For this review, take the finished solid that the model builds, in its own axes (mm). Face numbers are marked on the shaded views. A direction names the side the tool comes from. Give positions to 0.01 mm unless a question says otherwise; leave off trailing zeros. Order: outer loops, then holes, each group sorted by start corner. A loop starts at its lowest first (then second) coordinate and runs counter-clockwise, first axis right, second up.
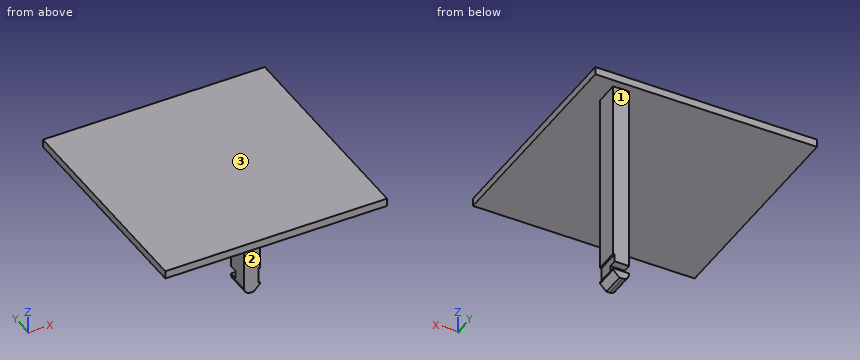
from build123d import *

# Parameters (mm, degrees)
F1_W      = 177.8
F1_H      = 177.8
F2_DEPTH  = 6.35
F3_W      = 12.7
F3_H      = 19.05
F4_DEPTH  = 165.1
F5_W      = 19.05
F5_H      = 12.7
F6_DEPTH  = 1.27
F7_SIZE   = 5.08
F8_R      = 5.08
F9_W      = 6.35
F9_H      = 6.35
F10_DEPTH = 25.4


with BuildPart() as f2:
    # F1 (on offset) → F2 (new body)
    with BuildSketch(Plane.XY.offset(177.8)):
        Rectangle(F1_W, F1_H)
    extrude(amount=F2_DEPTH)

    # F3 (on face) → F4 (join)
    with BuildSketch(Plane(origin=(0, 0, 177.8), x_dir=(1, 0, 0), z_dir=(0, 0, -1))):
        with Locations((64.77, -73.025)):
            Rectangle(F3_W, F3_H)
    extrude(amount=F4_DEPTH)

    # F5 (on face) → F6 (cut)
    with BuildSketch(Plane.YZ.offset(71.12)):
        with Locations((73.025, 25.4)):
            Rectangle(F5_W, F5_H)
    extrude(amount=-F6_DEPTH, mode=Mode.SUBTRACT)

    # F7
    f7_edges = [f2.edges().sort_by_distance(p)[0] for p in [
        (71.12, 73.025, 12.7),
    ]]
    chamfer(f7_edges, length=F7_SIZE)

    # F8
    f8_edges = [f2.edges().sort_by_distance(p)[0] for p in [
        (58.42, 73.025, 12.7),
    ]]
    fillet(f8_edges, radius=F8_R)

    # F9 (on face) → F10 (cut)
    with BuildSketch(Plane.YZ.offset(69.85)):
        with Locations((79.375, 22.225)):
            Rectangle(F9_W, F9_H)
    extrude(amount=-F10_DEPTH, mode=Mode.SUBTRACT)


solid = f2.part
1) Clearance check with flat-ended pins moving along their axes: pin 1 (1.5 mm diameter, centred on y = 69, z = 55.5, fed in from -X); pin 2 (7 mm diameter, centred on x = 68, z = 16.5, fed in from +Y); pin 3 (4 mm diameter, centred on x = 57.5, z = 151, fed in from -Y). State where each tip first meets the part, or that it passes through.
Answer sheet:
pin 1: stops at x = 58.42
pin 2: stops at y = 82.55
pin 3: stops at y = 63.5
2) We need section A-A on y = -77. Give the boundary of the cut face in (x, z).
Answer sheet:
outline: (-88.9, 177.8) - (88.9, 177.8) - (88.9, 184.15) - (-88.9, 184.15) - close
3) To check wall thickness, follow line 1 (Z direction, x = 59, y = -74); line 2 (X direction, y = 81, z = 53). State the ranges of each line that lie inside material, in increasing order.
Answer sheet:
line 1: z = 177.8 to 184.15
line 2: x = 58.42 to 71.12
4) Tool access review of the marked faces 1, 2 and 3: name each direction out of +Z, -Z, +X, -X, +Y, -Y from which nothing blocks a thin tool from reaching the whole face with its end or side.
Answer sheet:
face 1: -Z, +X, -X, +Y
face 2: -Z, +X, -X, -Y
face 3: +Z, +X, -X, +Y, -Y
5) We need section B-B on z = 34.5. Give the boundary of the cut face in (x, y).
Answer sheet:
outline: (58.42, 63.5) - (71.12, 63.5) - (71.12, 82.55) - (58.42, 82.55) - close
